Work out the finished part from the listing and answer in its coordinate system (mm). A direction names the side the tool comes from. Coordinates: 2 decimals unless noted, no trailing zeros. Order: outer loops, then holes, each group sorted by start corner. A loop starts at its lowest first (then second) coordinate and runs counter-clockwise, first axis right, second up. Notation, with made-up numbers: M -27.75,52.25 L -5.75,52.25 A20 cw -5.75,79.25 Z; hole C -13,8 d4. An arc over 180 degrees is marked long. Use a Markdown table: item, result. Add a question column.
Autodesk Inventor part; units mm, degrees
ref_plane "YZ Plane" through (0, 0, 0) normal (1, 0, 0) x (0, 1, 0)
ref_plane "XZ Plane" through (0, 0, 0) normal (0, 1, 0) x (-1, 0, 0)
ref_plane "XY Plane" through (0, 0, 0) normal (0, 0, 1) x (1, 0, 0)
sketch "Sketch1" plane through (0, 0, 0) normal (0, 0, 1) x (1, 0, 0)
  line L0 (-40, 7.5) -> (40, 7.5)
  line L1 (40, 7.5) -> (40, -7.5)
  line L2 (40, -7.5) -> (-40, -7.5)
  line L3 (-40, -7.5) -> (-40, 7.5)
  point P0 (0, 0)
  dimension "d0" = 80
  dimension "d1" = 15
  dimension "d2" = 40
  dimension "d3" = 7.5
extrude "Extrusion1" add sketch "Sketch1" along normal blind 2
sketch "Sketch2" plane through (0, 0, 2) normal (0, 0, 1) x (1, 0, 0)
  line L0 (-40, 7.5) -> (40, 7.5)
  line L1 (-40, -7.5) -> (-40, 7.5)
  arc A0 (-35, 2.5) -> (-35, -2.5) centre (-35, 0) ccw
  arc A1 (-25, -2.5) -> (-25, 2.5) centre (-25, 0) ccw
  line L2 (-35, 2.5) -> (-25, 2.5)
  line L3 (-25, -2.5) -> (-35, -2.5)
  arc A2 (25, 2.5) -> (25, -2.5) centre (25, 0) ccw
  arc A3 (35, -2.5) -> (35, 2.5) centre (35, 0) ccw
  line L4 (25, 2.5) -> (35, 2.5)
  line L5 (35, -2.5) -> (25, -2.5)
  point P0 (0, 0)
  dimension "d6" = 5
  dimension "d7" = 5
  dimension "d8" = 10
  dimension "d9" = 5
  dimension "d10" = 7.5
  dimension "d11" = 7.5
  dimension "d12" = 5
  dimension "d15" = 60
extrude "Extrusion2" cut sketch "Sketch2" against normal through all
fillet "Fillet1" radius 1 4 edges at (-40, 7.5, 1) (-40, -7.5, 1) (40, -7.5, 1) (40, 7.5, 1)
properties part number "SM-TM2" material "UHMW, White"
(1) A cutting plane is placed at B-B on y = -0.25. Write down the section's boundary in (x, z), plus the area to 3 significant figures.
(2) Which of the six approach directions +Z, -Z, +X, -X, +Y, -Y give full straight-line access (tool end or side, diameter ignored) to faces 1 (the cylindrical face through (22.5, 0.1, 1)), 2 (the flat face through (-1, 7.5, 1))?
(3) The mould has two halves that part along Y. Classify faces 3 (the flat face through (1, -7.5, 1)), 4 (the flat face through (-1, 0, 0)), 5 (the cylindrical face through (37.5, -0.1, 1)): pulls with the +Y half, pulls with the -Y half, needs draft (parallel to the pull), parting line crosses it, or undercut.
(4) Straight lines are drawn through the part: line 1 (X direction, y = 2, z = 1.95); line 2 (X direction, y = -1.75, z = 0.95); line 3 (Y direction, x = -36, z = 1). For each, find the intervals that lie inside material, in ascending order.
(5) A cutting plane is placed at A-A on z = 0.65. Write down the section's boundary in (x, y).
From the geometry:
| question | item | result |
|---|---|---|
| 1 | outline | M -40,0 L -37.49,0 L -37.49,2 L -40,2 Z; M -22.51,0 L 22.51,0 L 22.51,2 L -22.51,2 Z; M 37.49,0 L 40,0 L 40,2 L 37.49,2 Z |
| 1 | area | 100 mm2 |
| 2 | face 1 | +Z, -Z |
| 2 | face 2 | +Z, -Z, +X, -X, +Y |
| 3 | face 3 | pulls with the -Y half |
| 3 | face 4 | needs draft |
| 3 | face 5 | undercut |
| 4 | line 1 | x = -40 to -36.5, -23.5 to 23.5, 36.5 to 40 |
| 4 | line 2 | x = -40 to -36.79, -23.21 to 23.21, 36.79 to 40 |
| 4 | line 3 | y = -7.5 to -2.29, 2.29 to 7.5 |
| 5 | outline | M -40,-6.5 A1 ccw -39,-7.5 L 39,-7.5 A1 ccw 40,-6.5 L 40,6.5 A1 ccw 39,7.5 L -39,7.5 A1 ccw -40,6.5 Z; hole M -35,-2.5 L -25,-2.5 A2.5 ccw -25,2.5 L -35,2.5 A2.5 ccw Z; hole M 25,-2.5 L 35,-2.5 A2.5 ccw 35,2.5 L 25,2.5 A2.5 ccw Z |
